Work out the finished part from the listing and answer in its coordinate system (mm). Give positions to 0.01 mm unless a question says otherwise; leave off trailing zeros. Loops run counter-clockwise (first coordinate to the right, second up) from the corner with the lowest first, then second, coordinate; pieces in that order, holes last. Notation, with made-up numbers: (59, -29.75) - (101, -29.75) arc R13 ccw to (101, -8.75) - close; hole circle Ø5 at (9.5, 19.5). An arc over 180 degrees is marked (long way). One line per item, written item: value.
Autodesk Inventor part; units mm, degrees
ref_plane "YZ Plane" through (0, 0, 0) normal (1, 0, 0) x (0, 1, 0)
ref_plane "XZ Plane" through (0, 0, 0) normal (0, 1, 0) x (-1, 0, 0)
ref_plane "XY Plane" through (0, 0, 0) normal (0, 0, 1) x (1, 0, 0)
sketch "Sketch1" plane through (0, 0, 0) normal (0, 1, 0) x (-1, 0, 0)
  line L0 (-107.4651, -6.5728) -> (-108.712, 11.2585)
  arc A0 (-108.712, 11.2585) -> (-117.5803, 19.5283) centre (-117.5803, 10.6383) ccw
  line L1 (-117.5803, 19.5283) -> (-120.65, 19.5283)
  line L2 (-120.65, 19.5283) -> (-120.65, 24.13)
  arc A1 (-120.65, 24.13) -> (-118.2535, 38.6966) centre (-161.4319, 38.3198) ccw
  line L3 (-128.333, 181.8469) -> (-127, 193.5462)
  line L4 (-109.22, 203.2) -> (-7.62, 209.4141)
  arc A2 (-119.38, 167.7774) -> (-128.333, 181.8469) centre (-135.1274, 167.64) ccw
  line L5 (-107.4651, -6.5728) -> (0, 0)
  line L6 (-7.62, 209.4141) -> (0, 200.333)
  line L7 (0, 0) -> (0, 200.333)
  line L8 (-109.22, 203.2) -> (-127, 193.5462)
  line L9 (-118.2535, 38.6966) -> (-119.38, 167.7774)
  line L10 (0, 0) -> (-88.3844, 0) construction
  line L11 (-8.89, 7.0905) -> (-8.89, 184.8905) construction
  line L12 (-8.89, 7.0905) -> (-92.5537, 1.9734) construction
  line L13 (-114.808, 24.1003) -> (-115.616, 100.296) construction
  line L14 (-114.808, 24.1003) -> (-120.65, 186.0215) construction
  line L15 (32.2864, 0) -> (-193.7183, 0) construction
  line L16 (-38.1, 200.4246) -> (-90.8335, 197.1993) construction
  line L17 (-58.42, 206.3071) -> (-52.8471, 115.1911) construction
  point P0 (-50.7218, 4.532)
  point P1 (-8.89, 108.6905)
  point P2 (-8.89, 32.4905)
  dimension "d52" = 76.2
  dimension "d54" = 76.2
  dimension "d98" = 25
  dimension "d99" = 55
  dimension "d100" = 86.5
  dimension "d103" = 8.89
  dimension "d104" = 7.62
  dimension "d106" = 203.2
  dimension "d108" = 127
  dimension "d109" = 109.22
  dimension "d111" = 167.64
  dimension "d112" = 120.65
  dimension "d114" = 41.91
  dimension "d115" = 41.91
  dimension "d118" = 76.2
  dimension "d122" = 8.89
  dimension "d123" = 86
  dimension "d124" = 43.18
  dimension "d125" = 15.748
  dimension "d127" = 52.832
  dimension "d128" = 7.112
  dimension "d129" = 38.1
  dimension "d130" = 140
  dimension "d131" = 7.62
  dimension "d161" = 25.4
  dimension "d162" = 119.38
  dimension "d163" = 3
  dimension "d166" = 108.712
  dimension "d167" = 114.808
  dimension "d168" = 120.65
  dimension "d170" = 3.175
  dimension "d171" = 26.67
  dimension "d172" = 24.13
  dimension "d174" = 4.572
  dimension "d175" = 193.04
extrude "Plate1" add sketch "Sketch1" along normal blind 1.5875
fillet "Corner Round1" radius 3.175 9 edges at (0, 0.7937, 200.333) (7.62, 0.7937, 209.4141) (120.65, 0.7937, 24.13) (120.65, 0.7937, 19.5283) (107.4651, 0.7937, -6.5728) (127, 0.7937, 193.5462) (109.22, 0.7937, 203.2) (128.333, 0.7937, 181.8469) (0, 0.7937, 0)
hole "Hole1" at (8.89, 0, 184.8905) at (38.1, 0, 200.4246) at (90.8335, 0, 197.1993) at (120.65, 0, 186.0215) at (115.616, 0, 100.296) at (114.808, 0, 24.1003) at (50.7218, 0, 4.532) at (92.5537, 0, 1.9734) at (8.89, 0, 7.0905) at (8.89, 0, 108.6905) at (8.89, 0, 32.4905) direction (0, 1, 0) diameter 3.4544 end through all
equation "\"d60\" = Thickness"
equation "\"d49\" = Thickness"
equation "\"BendReliefWidth\" = Thickness"
equation "\"BendReliefDepth\" = 0.5 * Thickness"
equation "\"CornerReliefSize\" = 4 * Thickness"
equation "\"MinimumRemnant\" = 2 * Thickness"
equation "\"TransitionRadius\" = BendRadius"
equation "\"JacobiRadiusSize\" = BendRadius"
equation "\"GapSize\" = Thickness"
properties part number "J009859" material "POLYCARBONATE, CLEAR"
1. Section B-B (z = 123) is taken. Write down the section's boundary in (x, y).
Output:
outline: (0, 0) - (118.99, 0) - (118.99, 1.59) - (0, 1.59) - close
2. Find the intervals of material crossed by line 1 along Z through (x, y) = (8.89, 0.9); line 2 along Z through (x, y) = (39.5, 0.65); line 3 along X through (y, z) = (1.35, 116.5), in increasing order.
Output:
line 1: z = -0.54 to 5.36, 8.82 to 30.76, 34.22 to 106.96, 110.42 to 183.16, 186.62 to 209.32
line 2: z = -2.42 to 199.41, 201.44 to 207.46
line 3: x = 0 to 118.93
3. Section C-C (x = 76.5) is taken. Write down the section's boundary in (y, z).
Output:
outline: (0, -4.68) - (1.59, -4.68) - (1.59, 205.2) - (0, 205.2) - close
4. The mould has two halves that part along Z. Classify faces 1 (the cylindrical face through (121.4, 0.78, 175.36)), 2 (the flat face through (65, 0, 103)), 3 (the flat face through (59.562, 0.783, 206.237)), 4 (the cylindrical face through (111.56, 0.78, 17.18)): released by +Z, released by -Z, zero draft, split by the parting line, or undercut.
Output:
face 1: undercut
face 2: zero draft
face 3: released by +Z
face 4: released by -Z
5. Section A-A (y = 0.5) is taken. Count the separate pieces of the cut face and the enclosed holes in it, and give its area (3 significant figures).
Output:
separate pieces: 1
enclosed holes: 11
area: 24,700 mm²
